Part model, mm, in its own coordinate system. A direction names the side the tool comes from. Give positions to 0.01 mm unless a question says otherwise; leave off trailing zeros. Order: outer loops, then holes, each group sorted by start corner. A loop starts at its lowest first (then second) coordinate and runs counter-clockwise, first axis right, second up.
1. Mould opens along Y. For faces 3 (the cylindrical face through (0.1, -8.43, -1.4)), 4 (the flat face through (1.5, 0.585, 1.8)), 5 (the flat face through (-8, 0, 5)) say: +Y half, -Y half, draft (parallel to the pull), parting line (faces both ways), or undercut.
2. Slice it at A-A on z = 2.25. Give the number of separate pieces and of enclosed holes in the cut face, and give its area (3 significant figures).
3. Drop a flat-ended pin along its axis: pin 1 Ø4.5 at (x, y) = (-1, -0.5) entering from +Z. Give the stop position or say it passes through.
4. Which spindle directions (+Z, -Z, +X, -X, +Y, -Y) get a long thin tool onto all of the face, cutting with end or side? Do faces 1 (the flat face through (9, 0, 2)), 2 (the flat face through (2.05, 0, 2)). Say none if no direction does.
5. Probe line 1 (Y direction, x = 0, z = 2); line 2 (Y direction, x = -1.5, z = 0.75) (3 decimals); line 3 (X direction, y = -4.25, z = 2.75). List the from-to ranges inside material, lowest first.
6. Slice it at B-B on x = 0. List the corners of the cut face in (y, z), and give its area (3 significant figures).
7. Slice it at C-C on y = 3.5. List the corners of the cut face in (x, z), and give its area (3 significant figures).
from build123d import *

# Parameters (mm, degrees)
SKETCH1_W           = 18
SKETCH1_H           = 18
BOSS_EXTRUDE1_DEPTH = 2
SKETCH1_4_R         = 2.75
BOSS_EXTRUDE2_DEPTH = 4
SKETCH1_5_W         = 18
SKETCH1_5_H         = 18
SKETCH1_5_W_2       = 15
SKETCH1_5_H_2       = 15
BOSS_EXTRUDE3_DEPTH = 5
CHAMFER1_SIZE       = 0.3
FILLET3_R           = 0.3
FILLET4_R           = 2


with BuildPart() as part:
    # Sketch1 → Boss-Extrude1 (new body)
    with BuildSketch(Plane.XY):
        Rectangle(SKETCH1_W, SKETCH1_H)
    extrude(amount=-BOSS_EXTRUDE1_DEPTH)

    # Sketch1<4> → Boss-Extrude2 (add)
    with BuildSketch(Plane.XY):
        Circle(SKETCH1_4_R)
        Polygon((-0.585, 0.585), (-0.585, 2.05), (0.585, 2.05), (0.585, 0.585), (2.05, 0.585), (2.05, -0.585), (0.585, -0.585), (0.585, -2.05), (-0.585, -2.05), (-0.585, -0.585), (-2.05, -0.585), (-2.05, 0.585), align=None, mode=Mode.SUBTRACT)
    extrude(amount=BOSS_EXTRUDE2_DEPTH)

    # Sketch1<5> → Boss-Extrude3 (add)
    with BuildSketch(Plane.XY):
        Rectangle(SKETCH1_5_W, SKETCH1_5_H)
        Rectangle(SKETCH1_5_W_2, SKETCH1_5_H_2, mode=Mode.SUBTRACT)
    extrude(amount=BOSS_EXTRUDE3_DEPTH)

    # Chamfer1
    chamfer1_edges = [part.edges().sort_by_distance(p)[0] for p in [
        (1.3175, -0.585, 4),
        (0, -2.05, 4),
        (-0.585, -1.3175, 4),
        (-1.3175, -0.585, 4),
        (-2.05, 0, 4),
        (-0.585, 1.3175, 4),
        (1.3175, 0.585, 4),
        (2.05, 0, 4),
        (0.585, -1.3175, 4),
        (-1.3175, 0.585, 4),
        (0, 2.05, 4),
        (0.585, 1.3175, 4),
    ]]
    chamfer(chamfer1_edges, length=CHAMFER1_SIZE)

    # Fillet3
    fillet3_edges = [part.edges().sort_by_distance(p)[0] for p in [
        (0.585, 0.585, 1.85),
        (0.585, -0.585, 1.85),
        (-0.585, -0.585, 1.85),
        (-0.585, 0.585, 1.85),
    ]]
    fillet(fillet3_edges, radius=FILLET3_R)

    # Fillet4
    fillet4_edges = [part.edges().sort_by_distance(p)[0] for p in [
        (9, 0, -2),
        (0, 9, -2),
        (-9, 0, -2),
        (0, 7.5, 0),
        (-7.5, 7.5, 2.5),
        (7.5, 0, 0),
        (7.5, 7.5, 2.5),
        (7.5, -7.5, 2.5),
        (-7.5, -7.5, 2.5),
        (-7.5, 0, 0),
        (0, -7.5, 0),
        (0, -9, -2),
        (-9, 9, 1.5),
        (9, 9, 1.5),
        (9, -9, 1.5),
        (-9, -9, 1.5),
    ]]
    fillet(fillet4_edges, radius=FILLET4_R)


solid = part.part
Data:
1. face 3: -Y half
1. face 4: undercut
1. face 5: draft
2. separate pieces: 2
2. enclosed holes: 2
2. area: 114 mm2
3. pin 1: stops at z = 4
4. face 1: +Z, -Z, +X, +Y, -Y
4. face 2: +Z
5. line 1: y = -9 to -7.5, -2.75 to -2.05, 2.05 to 2.75, 7.5 to 9
5. line 2: y = -9 to -7.061, -2.305 to -0.585, 0.585 to 2.305, 7.061 to 9
5. line 3: x = -9 to -7.5, 7.5 to 9
6. outline: (-9, 0) arc R2 ccw to (-7, -2) - (7, -2) arc R2 ccw to (9, 0) - (9, 5) - (7.5, 5) - (7.5, 2) arc R2 cw to (5.5, 0) - (2.75, 0) - (2.75, 4) - (2.35, 4) - (2.05, 3.7) - (2.05, 0) - (-2.05, 0) - (-2.05, 3.7) - (-2.35, 4) - (-2.75, 4) - (-2.75, 0) - (-5.5, 0) arc R2 cw to (-7.5, 2) - (-7.5, 5) - (-9, 5) - close
6. area: 56.5 mm2
7. outline: (-9, 0) arc R2 ccw to (-7, -2) - (7, -2) arc R2 ccw to (9, 0) - (9, 5) - (7.5, 5) - (7.5, 2) arc R2 cw to (5.5, 0) - (-5.5, 0) arc R2 cw to (-7.5, 2) - (-7.5, 5) - (-9, 5) - close
7. area: 51.0 mm2
